Autodesk Inventor part; units mm, degrees
ref_plane "Work Plane1" through (0, 0, 5.5753) normal (0, 0, 1) x (1, 0, 0)
ref_plane "YZ Plane" through (0, 0, 0) normal (1, 0, 0) x (0, 1, 0)
ref_plane "XZ Plane" through (0, 0, 0) normal (0, 1, 0) x (-1, 0, 0)
sketch "Sketch1" plane through (0, 0, 0) normal (0, 0, 1) x (1, 0, 0)
  circle A0 centre (0, 0) radius 2.3813 construction
  line L0 (1.3748, 2.3813) -> (2.7496, 0)
  line L1 (2.7496, 0) -> (1.3748, -2.3812)
  line L2 (1.3748, -2.3812) -> (-1.3748, -2.3813)
  line L3 (-1.3748, -2.3813) -> (-2.7496, 0)
  line L4 (-2.7496, 0) -> (-1.3748, 2.3812)
  line L5 (-1.3748, 2.3812) -> (1.3748, 2.3813)
  point P0 (0, 2.3813)
  dimension "d0" = 4.7625
extrude "Extrusion1" add sketch "Sketch1" along normal blind 0.8128
sketch "Sketch2" plane through (0, 0, 0.8128) normal (0, 0, 1) x (1, 0, 0)
  circle A0 centre (0, 0) radius 1.0795
  dimension "d3" = 2.159
extrude "Extrusion2" add sketch "Sketch2" along normal blind 3.175
sketch "Sketch3" plane through (0, 0, 3.9878) normal (0, 0, 1) x (1, 0, 0)
  circle A0 centre (0, 0) radius 1.0795
  circle A1 centre (0, 0) radius 2.0637
  line L0 (0, 2.0637) -> (0, -2.0637)
  dimension "d6" = 4.1275
revolve "Revolution1" add sketch "Sketch3" angle 360 about axis through (0, 2.0637, 3.9878) along (0, -1, 0) picked at (-0.2386, -0.2693) picked at (-0.2507, -1.7052) contours L0 A0 | A0 L0 A1
fillet "Fillet1" radius 0.381 2 edges at (-1.0795, 0, 0.8128) (-1.0795, 0, 2.2289)
ref_plane "Work Plane1" through (0, 0, 5.5753) normal (0, 0, 1) x (1, 0, 0)
split "Split1" plane through (0, 0, 5.5753) removes the side toward (0, 0, 1)
sketch "Sketch4" plane through (0, 0, 0) normal (0, 0, -1) x (-1, 0, 0)
  circle A0 centre (0, 0) radius 1.2329
  circle A1 centre (0, 0) radius 1.4224
  dimension "d10" = 2.8448
extrude "Extrusion3" add sketch "Sketch4" along normal blind 9.525 contours A0 | A1
chamfer "Chamfer1" distance 0.381 angle 45 1 edges at (1.4224, 0, -9.525)
thread "Thread1"
properties part number "0.1875 Ball Stud 0.375"
Work out the finished part from the listing and answer in its coordinate system (mm). A direction names the side the tool comes from. Coordinates: 2 decimals unless noted, no trailing zeros. Loops run counter-clockwise (first coordinate to the right, second up) from the corner with the lowest first, then second, coordinate; pieces in that order, holes last.
1) Section A-A (z = -4) is taken. Give the vertices of the cut face in (x, y), plus the area to 3 significant figures.
Results:
outline: circle Ø2.84 at (0, 0)
area: 6.36 mm2
2) For a pull along Z with two mould halves and no side action, classify faces 1 (the flat face through (2.072, -1.174, 0.401)), 2 (the flat face through (1.2, 1.1, 0)), 3 (the flat face through (1.2, 1.1, 0.813)) as +Z half, -Z half, draft (parallel to the pull), parting line (faces both ways), or undercut.
Results:
face 1: draft
face 2: -Z half
face 3: undercut
3) Consider probe 1 along Z at (x, y) = (0.8, -1.95); probe 2 along Z at (x, y) = (1.8, 0.2); probe 3 along Z at (x, y) = (-1.6, 1). Determine where each line is inside the solid, lowest interval first.
Results:
probe 1: z = 0 to 0.81
probe 2: z = 0 to 0.81, 3 to 4.98
probe 3: z = 0 to 0.81, 3.15 to 4.82
4) Flat-ended cylindrical pins translate along their axes: pin 1 (1 mm diameter, centred on y = 1.5, z = 4.5, fed in from -X); pin 2 (2 mm diameter, centred on y = 0.5, z = -3, fed in from -X). Find the tip coordinate at first contact, or state that the pin passes through.
Results:
pin 1: stops at x = -1.76
pin 2: stops at x = -1.42
5) For faces 4 (the cylindrical face through (0.31, 1.39, -4.51)), 5 (the flat face through (-2.072, 1.174, 0.401)), 6 (the cylindrical face through (-0.14, -1.07, 1.6)), determine the directions among +Z, -Z, +X, -X, +Y, -Y from which every point of the face is accessible in a straight line to the end or side of a thin tool.
Results:
face 4: -Z
face 5: +Z, -Z, -X, +Y
face 6: none
